Geometry check sheet. Reference: the model listing, model coordinates, mm. Face numbers are marked on the shaded views. Coordinates: 2 decimals unless noted, no trailing zeros. Order: outer loops, then holes, each group sorted by start corner. A loop starts at its lowest first (then second) coordinate and runs counter-clockwise, first axis right, second up. Notation, with made-up numbers: M -36.5,12 L 16.5,12 A7 ccw 16.5,24 Z; hole C -18.75,10.5 d5. An arc over 180 degrees is marked long. One line per item, written item: value. Start each with the question number.
1) Sectioned sample at D-D, the plane z = 11.75. Enter the section's corners in (x, y).
2) Sectioned sample at C-C, the plane x = -39.5. Enter the section's corners in (y, z).
3) Thickness scan on L1, parallel to X at y = 1.5, z = 7.75; L2, parallel to Y at x = 0, z = 4; L3, parallel to X at y = -40, z = 8.5. Record the ranges inside material, lowest first. Write a range as from..to.
4) Sectioned sample at B-B, the plane z = 3. Enter the section's corners in (x, y), then the cut area to 3 significant figures.
5) Sectioned sample at A-A, the plane x = 0. Enter the section's corners in (y, z).
6) Go/stop test with flat-tipped pins: P1, Ø2, axis at x = 28.5, z = 9.5, coming from the -Y side; P2, Ø8, axis at y = -10.5, z = 3.5, coming from the +X side; P3, Ø2, axis at y = 28.5, z = 13, coming from the -X side; P4, Ø2, axis at x = 39.5, y = -23.5, coming from the +Z side. Record where each tip stops, or that it passes through.
7) Draft check along Y on the marked faces 1, 2 and 3. Enter one of: pulls with the +Y half, pulls with the -Y half, needs draft (parallel to the pull), parting line crosses it, or undercut.
Solid Edge part; units mm, degrees
sketch "Sketch1" plane through (0, 0, 0) normal (0, 0, 1) x (1, 0, 0)
  circle A0 centre (0, 0) radius 47.5
  circle A1 centre (0, 0) radius 54.5
extrude "Protrusion1" add sketch "Sketch1" along normal blind 15
sketch "Sketch2" plane through (0, 0, 0) normal (1, 0, 0) x (0, 1, 0)
  line L0 (-3.3486, 7.7174) -> (-1.6743, 10.6174)
  line L1 (-1.6743, 4.8174) -> (-3.3486, 7.7174)
  line L2 (1.6743, 4.8174) -> (-1.6743, 4.8174)
  line L3 (3.3486, 7.7174) -> (1.6743, 4.8174)
  line L4 (1.6743, 10.6174) -> (3.3486, 7.7174)
  line L5 (0, 13.5174) -> (1.6743, 10.6174)
  line L6 (-1.6743, 10.6174) -> (0, 13.5174)
extrude "ExtrudedCutout_1" cut sketch "Sketch2" along normal mid plane 104
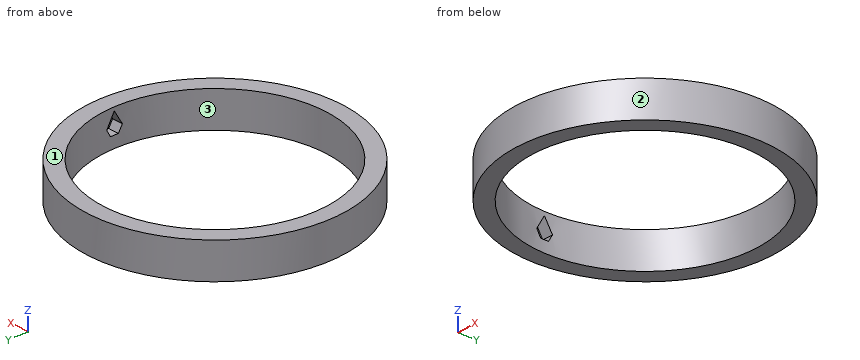
Final values:
1. outline: C 0,0 d109; hole M -52,-1.02 L -47.49,-1.02 A47.5 ccw 47.49,-1.02 L 52,-1.02 L 52,1.02 L 47.49,1.02 A47.5 ccw -47.49,1.02 L -52,1.02 Z
2. outline: M -37.55,0 L -26.38,0 L -26.38,15 L -37.55,15 Z; M 26.38,0 L 37.55,0 L 37.55,15 L 26.38,15 Z
3. L1: x = -54.48..-52, 52..54.48
3. L2: y = -54.5..-47.5, 47.5..54.5
3. L3: x = -37.02..-25.62, 25.62..37.02
4. outline: C 0,0 d109; hole C 0,0 d95
4. area: 2,240 mm^2
5. outline: M -54.5,0 L -47.5,0 L -47.5,15 L -54.5,15 Z; M 47.5,0 L 54.5,0 L 54.5,15 L 47.5,15 Z
6. P1: stops at y = -47.05
6. P2: stops at x = 54.11
6. P3: stops at x = -47.05
6. P4: passes through
7. face 1: needs draft
7. face 2: parting line crosses it
7. face 3: undercut
